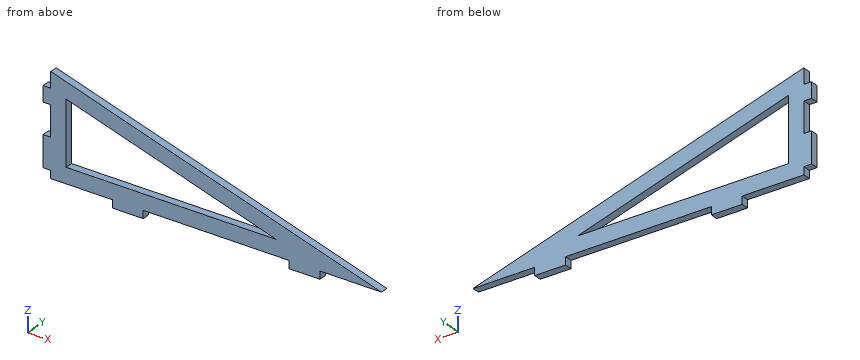
```python
from build123d import *

# Parameters (mm, degrees)
BOSS_EXTRUDE1_DEPTH = 3.175


with BuildPart() as part:
    # Sketch1 → Boss-Extrude1 (new body)
    with BuildSketch(Plane(origin=(0, 0, 0), x_dir=(1, 0, 0), z_dir=(0, 1, 0))):
        Polygon((68.1228, 20.51), (42.7228, 20.51), (42.7228, 23.685), (30.0228, 23.685), (30.0228, 20.51), (-30.0228, 20.51), (-30.0228, 23.685), (-42.7228, 23.685), (-42.7228, 20.51), (-68.1228, 20.51), (-68.1228, 17.335), (-71.2978, 17.335), (-71.2978, 4.635), (-68.1228, 4.635), (-68.1228, -7.81), (-71.2978, -7.81), (-71.2978, -14.16), (-68.1228, -14.16), (-68.1228, -20.51), align=None)
        Polygon((-61.7728, 14.16), (-61.7728, -11.966623033), (25.00529437, 14.16), align=None, mode=Mode.SUBTRACT)
    extrude(amount=BOSS_EXTRUDE1_DEPTH)


solid = part.part
```
The listing builds one solid part. Answer for the finished solid, in the listing's coordinates (mm). Round coordinates to 2 decimals unless told otherwise and drop trailing zeros. Write each loop counter-clockwise with the first axis right and the second up, starting at its lowest first coordinate (ties: lowest second). Pieces come first, ordered by that corner, then holes. Notation, with made-up numbers: (50.5, 46.5) -> (94.5, 46.5) arc R29 cw to (94.5, 76.5) -> close; hole circle Ø5 at (26, 4). An arc over 180 degrees is marked (long way). Answer as a JSON object with one key per item and string values. Group by question number.
Q1. Each of these flat-tipped pins is pushed along its axis until it touches: pin 1 Ø1 at (x, y) = (-69.5, 2.5) entering from -Z (3 decimals); pin 2 Ø1.6 at (x, y) = (-18, 1) entering from +Z; pin 3 Ø1 at (x, y) = (13, 2) entering from -Z. Where does it stop, or does it pass through?
Q2. Straight lines are drawn through the part: line 1 along Z through (x, y) = (-26, 0.55); line 2 along Z through (x, y) = (-21.5, 1.4); line 3 along Z through (x, y) = (56, 0.7). For each, find the intervals that lie inside material, in ascending order.
Q3. Section A-A (y = 2.6) is taken. Write down the section's boundary in (x, z) (3 decimals), plus the area to 3 significant figures.
Q4. Section C-C (x = -6.5) is taken. Write down the section's boundary in (y, z) (3 decimals).
Q5. Section B-B (z = 2) is taken. Write down the section's boundary in (x, y) (3 decimals), plus the area to 3 significant figures.
Check values:
{
 "1": {"pin 1": "z = -17.335", "pin 2": "z = 5.66", "pin 3": "z = -20.51"},
 "2": {"line 1": "-20.51 to -14.16, 1.2 to 7.83", "line 2": "-20.51 to -14.16, -0.16 to 6.47", "line 3": "-20.51 to -16.86"},
 "3": {"outline": "(-71.298, -17.335) -> (-68.123, -17.335) -> (-68.123, -20.51) -> (-42.723, -20.51) -> (-42.723, -23.685) -> (-30.023, -23.685) -> (-30.023, -20.51) -> (30.023, -20.51) -> (30.023, -23.685) -> (42.723, -23.685) -> (42.723, -20.51) -> (68.123, -20.51) -> (-68.123, 20.51) -> (-68.123, 14.16) -> (-71.298, 14.16) -> (-71.298, 7.81) -> (-68.123, 7.81) -> (-68.123, -4.635) -> (-71.298, -4.635) -> close; hole (-61.773, -14.16) -> (25.005, -14.16) -> (-61.773, 11.967) -> close", "area": "1,800 mm^2"},
 "4": {"outline": "(0, -20.51) -> (3.175, -20.51) -> (3.175, -14.16) -> (0, -14.16) -> close; (0, -4.675) -> (3.175, -4.675) -> (3.175, 1.957) -> (0, 1.957) -> close"},
 "5": {"outline": "(-68.123, 0) -> (-61.773, 0) -> (-61.773, 3.175) -> (-68.123, 3.175) -> close; (-28.669, 0) -> (-6.643, 0) -> (-6.643, 3.175) -> (-28.669, 3.175) -> close", "area": "90.1 mm^2"}
}
